Geometry check sheet. Reference: the model listing, model coordinates, mm. Round coordinates to 2 decimals unless told otherwise and drop trailing zeros. Order: outer loops, then holes, each group sorted by start corner. A loop starts at its lowest first (then second) coordinate and runs counter-clockwise, first axis right, second up. Notation, with made-up numbers: M 18,18 L 46,18 A24 ccw 46,53 Z; hole C -39.75,0 d2. An arc over 180 degrees is marked long. Return JSON: item names as keys, results as strings. Group by question number.
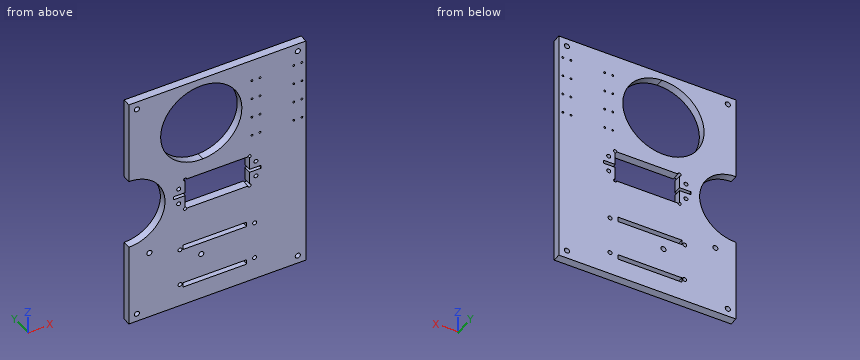
```python
from build123d import *

# Parameters (mm, degrees)
SKETCH_1_R         = 0.6
SKETCH_1_R_2       = 1.6
SKETCH_1_W         = 39.63
SKETCH_1_H         = 3
EXTRUDE_1_DEPTH    = 5
HOLE_WIZARD_M3_1_D = 2.5


with BuildPart() as part:
    # 草圖1 → 填料-伸長1 (new body)
    with BuildSketch(Plane(origin=(0, 0, 0), x_dir=(1, 0, 0), z_dir=(0, 1, 0))):
        with BuildLine():
            Line((110, 75), (0, 75))
            Line((0, 75), (0, 22.5))
            ThreePointArc((0, 22.5), (22.5, 0), (0, -22.5))
            Line((0, -22.5), (0, -75))
            Line((0, -75), (46, -75))
            Line((46, -75), (110, -75))
            Line((110, -75), (110, 75))
        make_face()
        with Locations(Location((76.5, -61.25, 0), (0, 0, 270))):
            Circle(SKETCH_1_R, mode=Mode.SUBTRACT)
        with Locations(Location((5, 70, 0), (0, 0, 270))):
            Circle(SKETCH_1_R_2, mode=Mode.SUBTRACT)
        with Locations(Location((5, -70, 0), (0, 0, 270))):
            Circle(SKETCH_1_R_2, mode=Mode.SUBTRACT)
        with Locations(Location((105, -70, 0), (0, 0, 270))):
            Circle(SKETCH_1_R_2, mode=Mode.SUBTRACT)
        with Locations(Location((105, 70, 0), (0, 0, 270))):
            Circle(SKETCH_1_R_2, mode=Mode.SUBTRACT)
        with Locations(Location((107.5, -61.25, 0), (0, 0, 270))):
            Circle(SKETCH_1_R, mode=Mode.SUBTRACT)
        with Locations(Location((107.5, -48.75, 0), (0, 0, 270))):
            Circle(SKETCH_1_R, mode=Mode.SUBTRACT)
        with Locations(Location((102.5, -48.75, 0), (0, 0, 270))):
            Circle(SKETCH_1_R, mode=Mode.SUBTRACT)
        with Locations(Location((107.5, -23.75, 0), (0, 0, 270))):
            Circle(SKETCH_1_R, mode=Mode.SUBTRACT)
        with Locations(Location((102.5, -36.25, 0), (0, 0, 270))):
            Circle(SKETCH_1_R, mode=Mode.SUBTRACT)
        with Locations(Location((81.5, -48.75, 0), (0, 0, 270))):
            Circle(SKETCH_1_R, mode=Mode.SUBTRACT)
        with Locations(Location((102.5, -23.75, 0), (0, 0, 270))):
            Circle(SKETCH_1_R, mode=Mode.SUBTRACT)
        with Locations(Location((107.5, -36.25, 0), (0, 0, 270))):
            Circle(SKETCH_1_R, mode=Mode.SUBTRACT)
        with Locations(Location((102.5, -61.25, 0), (0, 0, 270))):
            Circle(SKETCH_1_R, mode=Mode.SUBTRACT)
        with Locations(Location((81.5, -36.25, 0), (0, 0, 270))):
            Circle(SKETCH_1_R, mode=Mode.SUBTRACT)
        with Locations(Location((76.5, -48.75, 0), (0, 0, 270))):
            Circle(SKETCH_1_R, mode=Mode.SUBTRACT)
        with Locations(Location((81.5, -61.25, 0), (0, 0, 270))):
            Circle(SKETCH_1_R, mode=Mode.SUBTRACT)
        with Locations(Location((81.5, -23.75, 0), (0, 0, 270))):
            Circle(SKETCH_1_R, mode=Mode.SUBTRACT)
        with Locations(Location((76.5, -36.25, 0), (0, 0, 270))):
            Circle(SKETCH_1_R, mode=Mode.SUBTRACT)
        with Locations(Location((76.5, -23.75, 0), (0, 0, 270))):
            Circle(SKETCH_1_R, mode=Mode.SUBTRACT)
        with Locations(Location((45, 45, 0), (0, 0, 270))):
            Circle(SKETCH_1_R_2, mode=Mode.SUBTRACT)
        with Locations(Location((12.75503676, 31.388888889, 0), (0, 0, 270))):
            Circle(SKETCH_1_R_2, mode=Mode.SUBTRACT)
        with BuildLine():
            Line((75, -9), (75, -1))
            Line((75, -1), (82.2, -1))
            Line((82.2, -1), (82.2, 1))
            Line((82.2, 1), (75, 1))
            Line((75, 1), (75, 9))
            ThreePointArc((75, 9), (75.707106781, 10.707106781), (74, 10))
            Line((74, 10), (36, 10))
            ThreePointArc((36, 10), (34.292893219, 10.707106781), (35, 9))
            Line((35, 9), (35, 1))
            Line((35, 1), (27.8, 1))
            Line((27.8, 1), (27.8, -1))
            Line((27.8, -1), (35, -1))
            Line((35, -1), (35, -9))
            ThreePointArc((35, -9), (34.292893219, -10.707106781), (36, -10))
            Line((36, -10), (74, -10))
            ThreePointArc((74, -10), (75.707106781, -10.707106781), (75, -9))
        make_face(mode=Mode.SUBTRACT)
        with Locations((53.375, 61.625)):
            Rectangle(SKETCH_1_W, SKETCH_1_H, mode=Mode.SUBTRACT)
        with Locations((53.375, 35.875)):
            Rectangle(SKETCH_1_W, SKETCH_1_H, mode=Mode.SUBTRACT)
        with BuildLine():
            ThreePointArc((46, -70.230190249), (70.25, -45), (46, -19.769809751))
            ThreePointArc((46, -19.769809751), (19.75, -45), (46, -70.230190249))
        make_face(mode=Mode.SUBTRACT)
    extrude(amount=-EXTRUDE_1_DEPTH)

    # M3 螺紋孔1 (through all)
    with Locations(Plane(origin=(0, 0, 0), x_dir=(1, 0, 0), z_dir=(0, 1, 0))):
        with Locations((31, 5), (31, -5), (79, -5), (79, 5), (31.81, 36.875), (31.81, 60.625), (78.19, 60.625), (78.19, 36.875)):
            Hole(HOLE_WIZARD_M3_1_D / 2)


solid = part.part
```
Q1. Material ranges on line 1 along Z through (x, y) = (81.5, -3.45); line 2 along Z through (x, y) = (102.5, -2.9); line 3 along X through (y, z) = (-1.55, -70), recorded low to high.
Q2. Section check B-B on x = 56. Record the cut outline in (y, z) (3 decimals).
Q3. Section check A-A on z = 64. Record the cut outline in (x, y).
Q4. Depth check by flat-ended pin: pin 1 Ø2 at (x, z) = (31.81, -60.625) entering from +Y; pin 2 Ø8 at (x, z) = (72.5, 58) entering from +Y. Enter the tip coordinate at first touch or a pass-through.
Q5. Section check C-C on y = -1.1. Count the separate pieces of the cut face and the enclosed holes in it, plus the area to 3 significant figures.
Q6. Section check D-D on z = 14. Record the cut outline in (x, y).
Geometry check:
{
 "1": {"line 1": "z = -75 to -1, 1 to 23.15, 24.35 to 35.65, 36.85 to 48.15, 49.35 to 60.65, 61.85 to 75", "line 2": "z = -75 to 23.15, 24.35 to 35.65, 36.85 to 48.15, 49.35 to 60.65, 61.85 to 75", "line 3": "x = 0 to 3.4, 6.6 to 103.4, 106.6 to 110"},
 "2": {"outline": "M -5,-75 L 0,-75 L 0,-63.125 L -5,-63.125 Z; M -5,-60.125 L 0,-60.125 L 0,-37.375 L -5,-37.375 Z; M -5,-34.375 L 0,-34.375 L 0,-10 L -5,-10 Z; M -5,10 L 0,10 L 0,22.272 L -5,22.272 Z; M -5,67.728 L 0,67.728 L 0,75 L -5,75 Z"},
 "3": {"outline": "M 0,-5 L 28.37,-5 L 28.37,0 L 0,0 Z; M 61.63,-5 L 110,-5 L 110,0 L 61.63,0 Z"},
 "4": {"pin 1": "passes through", "pin 2": "stops at y = 0"},
 "5": {"separate pieces": "1", "enclosed holes": "34", "area": "12,500 mm^2"},
 "6": {"outline": "M 17.61,-5 L 110,-5 L 110,0 L 17.61,0 Z"}
}
